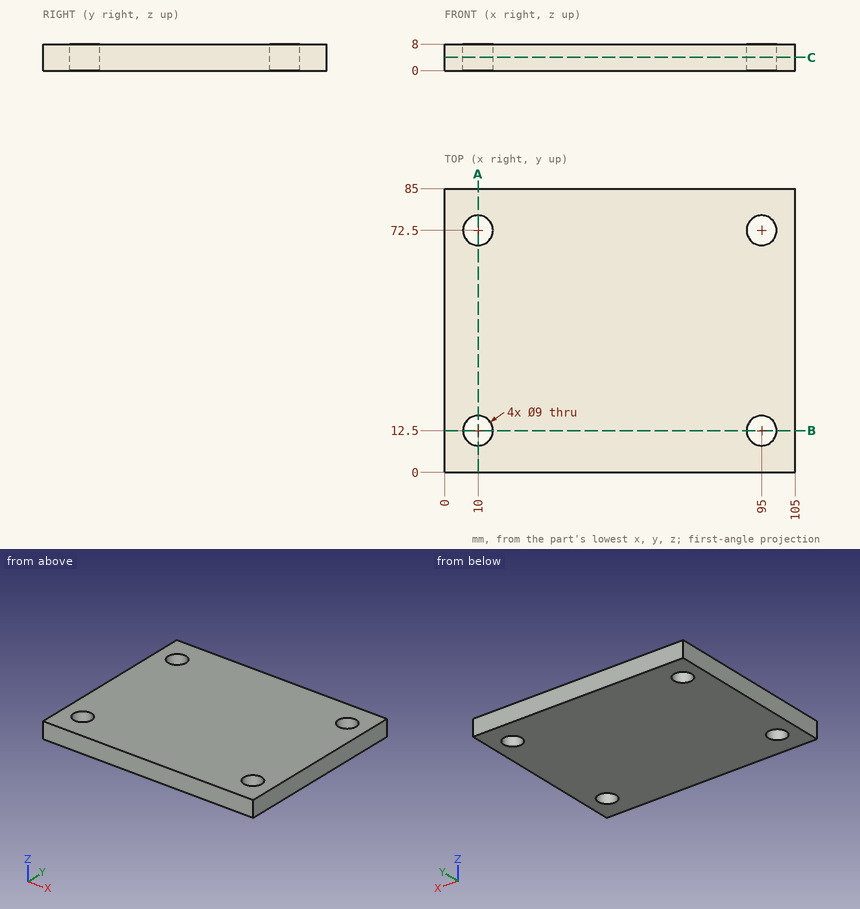
Source: three-view drawing plus pictorial views. Frame: mm from the lowest corner of the part. Coordinates: 2 decimals unless noted, no trailing zeros. Order: outer loops, then holes, each group sorted by start corner. A loop starts at its lowest first (then second) coordinate and runs counter-clockwise, first axis right, second up. Notation, with made-up numbers: M 64,7.25 L 95,7.25 A26 ccw 95,34.25 Z; hole C -5,-33.75 d2. An arc over 180 degrees is marked long. Answer in a Markdown table with one row per item.
(1) Material intervals for line 1 (Y direction, x = 10, z = 6.25); line 2 (X direction, y = 12.5, z = 3.25); line 3 (X direction, y = 8.5, z = 7), sorted ascending. Write a range as [from, to].
Numbers:
| item | result |
|---|---|
| line 1 | y = [0, 8], [17, 68], [77, 85] |
| line 2 | x = [0, 5.5], [14.5, 90.5], [99.5, 105] |
| line 3 | x = [0, 7.94], [12.06, 92.94], [97.06, 105] |
(2) Section query C-C, the plane z = 4. Output: boundary loops of the cut face in (x, y).
Numbers:
| item | result |
|---|---|
| outline | M 0,0 L 105,0 L 105,85 L 0,85 Z; hole C 10,12.5 d9; hole C 10,72.5 d9; hole C 95,12.5 d9; hole C 95,72.5 d9 |
(3) Section query A-A, the plane x = 10. Output: boundary loops of the cut face in (y, z).
Numbers:
| item | result |
|---|---|
| outline | M 0,0 L 8,0 L 8,8 L 0,8 Z; M 17,0 L 68,0 L 68,8 L 17,8 Z; M 77,0 L 85,0 L 85,8 L 77,8 Z |
(4) Section query B-B, the plane y = 12.5. Output: boundary loops of the cut face in (x, z).
Numbers:
| item | result |
|---|---|
| outline | M 0,0 L 5.5,0 L 5.5,8 L 0,8 Z; M 14.5,0 L 90.5,0 L 90.5,8 L 14.5,8 Z; M 99.5,0 L 105,0 L 105,8 L 99.5,8 Z |
